from build123d import *

# Parameters (mm, degrees)
SKETCH_1_W          = 86
SKETCH_1_H          = 86
EXTRUDE_1_DEPTH     = 50
SKETCH_2_R          = 40
EXTRUDE_2_DEPTH     = 86.5
SKETCH_3_R          = 30
EXTRUDE_3_DEPTH     = 3
SKETCH_4_R          = 12.5
EXTRUDE_4_DEPTH     = 4
SKETCH_5_R          = 10
EXTRUDE_5_DEPTH     = 36
SKETCH_7_W          = 6
SKETCH_7_H          = 25
EXTRUDE_6_DEPTH     = 12.5
SKETCH_8_R          = 36.5
CUT_EXTRUDE_1_DEPTH = 5
SKETCH_9_R          = 6.35
CUT_EXTRUDE_2_DEPTH = 30
SKETCH_10_R         = 2.1
CUT_EXTRUDE_3_DEPTH = 15
CHAMFER_1_SIZE      = 5
SKETCH_11_R         = 2.55
CUT_EXTRUDE_4_DEPTH = 15


with BuildPart() as part:
    # 草图1 → 凸台-拉伸1 (new body)
    with BuildSketch(Plane.XY):
        Rectangle(SKETCH_1_W, SKETCH_1_H)
    extrude(amount=EXTRUDE_1_DEPTH)

    # 草图2 → 凸台-拉伸2 (add)
    with BuildSketch(Plane.XY.offset(50)):
        Circle(SKETCH_2_R)
    extrude(amount=EXTRUDE_2_DEPTH)

    # 草图3 → 凸台-拉伸3 (add)
    with BuildSketch(Plane.XY.offset(136.5)):
        Circle(SKETCH_3_R)
    extrude(amount=EXTRUDE_3_DEPTH)

    # 草图4 → 凸台-拉伸4 (add)
    with BuildSketch(Plane.XY.offset(139.5)):
        Circle(SKETCH_4_R)
    extrude(amount=EXTRUDE_4_DEPTH)

    # 草图5 → 凸台-拉伸5 (add)
    with BuildSketch(Plane.XY.offset(143.5)):
        Circle(SKETCH_5_R)
    extrude(amount=EXTRUDE_5_DEPTH)

    # 草图7 → 凸台-拉伸6 (add)
    with BuildSketch(Plane(origin=(0, 0, 0), x_dir=(1, 0, 0), z_dir=(0, 1, 0))):
        with Locations((0, -162)):
            Rectangle(SKETCH_7_W, SKETCH_7_H)
    extrude(amount=EXTRUDE_6_DEPTH)

    # 草图8 → 切除-拉伸1 (cut)
    with BuildSketch(Plane(origin=(0, 0, 0), x_dir=(-1, 0, 0), z_dir=(0, 0, -1))):
        Circle(SKETCH_8_R)
    extrude(amount=-CUT_EXTRUDE_1_DEPTH, mode=Mode.SUBTRACT)

    # 草图9 → 切除-拉伸2 (cut)
    with BuildSketch(Plane(origin=(0, 0, 5), x_dir=(-1, 0, 0), z_dir=(0, 0, -1))):
        Circle(SKETCH_9_R)
    extrude(amount=-CUT_EXTRUDE_2_DEPTH, mode=Mode.SUBTRACT)

    # 草图10 → 切除-拉伸3 (cut)
    with BuildSketch(Plane(origin=(0, 0, 0), x_dir=(-1, 0, 0), z_dir=(0, 0, -1))):
        with Locations((-35, 35)):
            Circle(SKETCH_10_R)
        with Locations((35, 35)):
            Circle(SKETCH_10_R)
        with Locations((35, -35)):
            Circle(SKETCH_10_R)
        with Locations((-35, -35)):
            Circle(SKETCH_10_R)
    extrude(amount=-CUT_EXTRUDE_3_DEPTH, mode=Mode.SUBTRACT)

    # 倒角1
    chamfer_1_edges = [part.edges().sort_by_distance(p)[0] for p in [
        (-43, 43, 25),
        (43, 43, 25),
        (43, -43, 25),
        (-43, -43, 25),
    ]]
    chamfer(chamfer_1_edges, length=CHAMFER_1_SIZE)

    # 草图11 → 切除-拉伸4 (cut)
    with BuildSketch(Plane.XY.offset(136.5)):
        with Locations((-24.748737342, 24.748737342)):
            Circle(SKETCH_11_R)
        with Locations((24.748737342, 24.748737342)):
            Circle(SKETCH_11_R)
        with Locations((24.748737342, -24.748737342)):
            Circle(SKETCH_11_R)
        with Locations((-24.748737342, -24.748737342)):
            Circle(SKETCH_11_R)
    extrude(amount=-CUT_EXTRUDE_4_DEPTH, mode=Mode.SUBTRACT)


solid = part.part
Input: part model. Units: mm. Frame: model coordinates. A direction names the side the tool comes from. Give positions to 0.01 mm unless a question says otherwise; leave off trailing zeros. Order: outer loops, then holes, each group sorted by start corner. A loop starts at its lowest first (then second) coordinate and runs counter-clockwise, first axis right, second up. Notation, with made-up numbers: (89.5, 76.5) -> (99.5, 76.5) arc R7 ccw to (99.5, 84.5) -> close; hole circle Ø6 at (-4.75, 45.25). An arc over 180 degrees is marked (long way). Use one line per item in the form item = value.
1) Section D-D, the plane z = 161.5. Return loops of the section in (x, y), and give its area (3 significant figures).
Response values:
outline = (-3, 9.54) arc R10 ccw (long way) to (3, 9.54) -> (3, 12.5) -> (-3, 12.5) -> close
area = 330 mm^2
2) Section C-C, the plane z = 98.5. Return loops of the section in (x, y), and give its area (3 significant figures).
Response values:
outline = circle Ø80 at (0, 0)
area = 5,030 mm^2
3) Line query: probe 1 along Z at (x, y) = (-26, -32.5); probe 2 along Z at (x, y) = (-5, -14.5); probe 3 along Z at (x, y) = (-1.5, 10). Output: solid intervals per line, ascending.
Response values:
probe_1 = 0 to 50
probe_2 = 5 to 139.5
probe_3 = 5 to 143.5, 149.5 to 174.5
4) Section B-B, the plane y = -15.5. Return loops of the section in (x, z).
Response values:
outline = (-43, 0) -> (-33.05, 0) -> (-33.05, 5) -> (33.05, 5) -> (33.05, 0) -> (43, 0) -> (43, 50) -> (36.87, 50) -> (36.87, 136.5) -> (25.69, 136.5) -> (25.69, 139.5) -> (-25.69, 139.5) -> (-25.69, 136.5) -> (-36.87, 136.5) -> (-36.87, 50) -> (-43, 50) -> close
5) Reachability of faces 4 (the flat face through (25, 25, 121.5)), 5 (the flat face through (0, 12.5, 162)), 6 (the flat face through (-35, -35, 15)) from +Z, -Z, +X, -X, +Y, -Y: full face, straight path, thin tool, end or side. Return the list, or none.
Response values:
face_4 = +Z
face_5 = +Z, +X, -X, +Y
face_6 = -Z
6) Mould query, pull axis Y, two halves, no side actions, for faces 1 (the flat face through (-15, -26.5, 136.5)), 2 (the cylindrical face through (36.666, -36.278, 7.395)), 3 (the flat face through (-1, -43, 25)). Classes: pulls with the +Y half, pulls with the -Y half, needs draft (parallel to the pull), parting line crosses it, or undercut.
Response values:
face_1 = needs draft
face_2 = undercut
face_3 = pulls with the -Y half
7) First-contact query: pin 1 Ø10 at (y, z) = (10, 131) entering from -X; pin 2 Ø6 at (x, y) = (-24, -31) entering from +Z; pin 3 Ø1.5 at (x, y) = (-0.5, 11) entering from -Z; pin 4 Ø4.5 at (x, y) = (-24.75, 24.75) entering from -Z. Flat tips, straight axial feed; report the tip coordinate or a pass-through.
Response values:
pin_1 = -39.69
pin_2 = 136.5
pin_3 = 5
pin_4 = 0
